```python
from build123d import *

# Parameters (mm, degrees)
SKETCH1_W                     = 444.26599996
SKETCH1_H                     = 47.498
BASE_FLANGE1_DEPTH            = 2.286
EDGE_FLANGE1_STRIP_W          = 11.144
EDGE_FLANGE1_STRIP_H          = 2.286
EDGE_FLANGE1_STRIP_CUT_DEPTH  = 25.4
EDGE_FLANGE1_RELIEF_W         = 12.287
EDGE_FLANGE1_RELIEF_H         = 1.143
EDGE_FLANGE1_RELIEF_CUT_DEPTH = 2.286
EDGE_FLANGE1_DEPTH            = 25.4
EDGE_FLANGE2_STRIP_W          = 11.144
EDGE_FLANGE2_STRIP_H          = 2.286
EDGE_FLANGE2_STRIP_CUT_DEPTH  = 25.4
EDGE_FLANGE2_RELIEF_W         = 12.287
EDGE_FLANGE2_RELIEF_H         = 1.143
EDGE_FLANGE2_RELIEF_CUT_DEPTH = 2.286
EDGE_FLANGE2_DEPTH            = 25.4
EDGE_FLANGE6_STRIP_W          = 11.144
EDGE_FLANGE6_STRIP_H          = 2.286
EDGE_FLANGE6_STRIP_CUT_DEPTH  = 444.26599996
EDGE_FLANGE6_DEPTH            = 444.26599996
SKETCH52_R                    = 3
CUT_EXTRUDE2_DEPTH            = 231.225159807
SKETCH53_R                    = 3
CUT_EXTRUDE3_DEPTH            = 450.771788169
SKETCH54_W                    = 20.32
SKETCH54_H                    = 3.286
CUT_EXTRUDE4_DEPTH            = 227.280796306
CUT_EXTRUDE6_DEPTH            = 227.280796306
CUT_EXTRUDE6_DEPTH_BACK       = 227.280796306
SKETCH57_W                    = 12.932384232
SKETCH57_H                    = 5.987852531
SKETCH57_W_2                  = 12.889095721
SKETCH57_H_2                  = 5.98785253
SKETCH57_W_3                  = 14.589217144
SKETCH57_H_3                  = 5.987852532
SKETCH57_W_4                  = 12.590694247
SKETCH57_H_4                  = 5.987852533
SKETCH57_W_5                  = 11.791285089
SKETCH57_H_5                  = 5.654723841


# Sheet-metal steps are written as plain solids
with BuildPart() as part:
    # Sketch1 → Base-Flange1 (new body)
    with BuildSketch(Plane.XY):
        Rectangle(SKETCH1_W, SKETCH1_H)
    extrude(amount=-BASE_FLANGE1_DEPTH)

    # Edge-Flange1 strip (across the edge) → Edge-Flange1 strip cut (cut)
    with BuildSketch(Plane(origin=(222.13299998, -12.7, 0), x_dir=(-1, 0, 0), z_dir=(0, 1, 0))):
        with Locations((-4.572, -1.143)):
            Rectangle(EDGE_FLANGE1_STRIP_W, EDGE_FLANGE1_STRIP_H)
    extrude(amount=EDGE_FLANGE1_STRIP_CUT_DEPTH, mode=Mode.SUBTRACT)

    # Edge-Flange1 relief (on the sheet) → Edge-Flange1 relief cut (cut)
    with BuildSketch(Plane(origin=(221.13299998, -12.7, 0), x_dir=(-1, 0, 0), z_dir=(0, 0, 1))):
        with Locations((-5.0005, 0.5715)):
            Rectangle(EDGE_FLANGE1_RELIEF_W, EDGE_FLANGE1_RELIEF_H)
        with Locations((-5.0005, -25.9715)):
            Rectangle(EDGE_FLANGE1_RELIEF_W, EDGE_FLANGE1_RELIEF_H)
    extrude(amount=-EDGE_FLANGE1_RELIEF_CUT_DEPTH, mode=Mode.SUBTRACT)

    # Edge-Flange1 section (across the edge) → Edge-Flange1 (add)
    with BuildSketch(Plane(origin=(222.13299998, -12.7, 0), x_dir=(-1, 0, 0), z_dir=(0, 1, 0))):
        with BuildLine():
            Line((-2.286, 1), (-2.286, 12.7))
            Line((-2.286, 12.7), (0, 12.7))
            Line((0, 12.7), (0, 1))
            ThreePointArc((0, 1), (0.292893219, 0.292893219), (1, 0))
            Line((1, 0), (1, -2.286))
            ThreePointArc((1, -2.286), (-1.323552883, -1.323552883), (-2.286, 1))
        make_face()
    extrude(amount=EDGE_FLANGE1_DEPTH)

    # Edge-Flange2 strip (across the edge) → Edge-Flange2 strip cut (cut)
    with BuildSketch(Plane(origin=(-222.13299998, 12.7, 0), x_dir=(1, 0, 0), z_dir=(0, -1, 0))):
        with Locations((-4.572, -1.143)):
            Rectangle(EDGE_FLANGE2_STRIP_W, EDGE_FLANGE2_STRIP_H)
    extrude(amount=EDGE_FLANGE2_STRIP_CUT_DEPTH, mode=Mode.SUBTRACT)

    # Edge-Flange2 relief (on the sheet) → Edge-Flange2 relief cut (cut)
    with BuildSketch(Plane(origin=(-221.13299998, 12.7, 0), x_dir=(1, 0, 0), z_dir=(0, 0, 1))):
        with Locations((-5.0005, 0.5715)):
            Rectangle(EDGE_FLANGE2_RELIEF_W, EDGE_FLANGE2_RELIEF_H)
        with Locations((-5.0005, -25.9715)):
            Rectangle(EDGE_FLANGE2_RELIEF_W, EDGE_FLANGE2_RELIEF_H)
    extrude(amount=-EDGE_FLANGE2_RELIEF_CUT_DEPTH, mode=Mode.SUBTRACT)

    # Edge-Flange2 section (across the edge) → Edge-Flange2 (add)
    with BuildSketch(Plane(origin=(-222.13299998, 12.7, 0), x_dir=(1, 0, 0), z_dir=(0, -1, 0))):
        with BuildLine():
            Line((-2.286, 1), (-2.286, 12.7))
            Line((-2.286, 12.7), (0, 12.7))
            Line((0, 12.7), (0, 1))
            ThreePointArc((0, 1), (0.292893219, 0.292893219), (1, 0))
            Line((1, 0), (1, -2.286))
            ThreePointArc((1, -2.286), (-1.323552883, -1.323552883), (-2.286, 1))
        make_face()
    extrude(amount=EDGE_FLANGE2_DEPTH)

    # Edge-Flange6 strip (across the edge) → Edge-Flange6 strip cut (cut)
    with BuildSketch(Plane(origin=(222.13299998, 23.749, 0), x_dir=(0, -1, 0), z_dir=(-1, 0, 0))):
        with Locations((-4.572, -1.143)):
            Rectangle(EDGE_FLANGE6_STRIP_W, EDGE_FLANGE6_STRIP_H)
    extrude(amount=EDGE_FLANGE6_STRIP_CUT_DEPTH, mode=Mode.SUBTRACT)

    # Edge-Flange6 section (across the edge) → Edge-Flange6 (add)
    with BuildSketch(Plane(origin=(222.13299998, 23.749, 0), x_dir=(0, -1, 0), z_dir=(-1, 0, 0))):
        with BuildLine():
            Line((-2.286, 1), (-2.286, 12.7))
            Line((-2.286, 12.7), (0, 12.7))
            Line((0, 12.7), (0, 1))
            ThreePointArc((0, 1), (0.292893219, 0.292893219), (1, 0))
            Line((1, 0), (1, -2.286))
            ThreePointArc((1, -2.286), (-1.323552883, -1.323552883), (-2.286, 1))
        make_face()
    extrude(amount=EDGE_FLANGE6_DEPTH)

    # Sketch52 → Cut-Extrude2 (cut, through all)
    with BuildSketch(Plane(origin=(0, 26.035, 0), x_dir=(1, 0, 0), z_dir=(0, 1, 0))):
        with Locations(Location((120.65, -6.85, 0), (0, 0, 270))):
            Circle(SKETCH52_R)
        with Locations(Location((-120.65, -6.85, 0), (0, 0, 270))):
            Circle(SKETCH52_R)
    extrude(amount=-CUT_EXTRUDE2_DEPTH, mode=Mode.SUBTRACT)

    # Sketch53 → Cut-Extrude3 (cut, through all)
    with BuildSketch(Plane(origin=(224.41899998, 0, 0), x_dir=(0, 0, -1), z_dir=(1, 0, 0))):
        with Locations((-6.85, 0)):
            Circle(SKETCH53_R)
    extrude(amount=-CUT_EXTRUDE3_DEPTH, mode=Mode.SUBTRACT)

    # Sketch54 → Cut-Extrude4 (cut, symmetric)
    with BuildSketch(Plane.XY):
        Polygon((222.13299998, 13.843), (222.13299998, 18.296), (201.81299998, 18.296), (201.81299998, 13.216), (219.98999998, 13.216), (219.98999998, 13.843), align=None)
        with Locations((211.97299998, 24.392)):
            Rectangle(SKETCH54_W, SKETCH54_H)
    cut_extrude4 = extrude(amount=CUT_EXTRUDE4_DEPTH, both=True, mode=Mode.SUBTRACT)

    # Mirror1: Cut-Extrude4 across plane
    add(cut_extrude4.mirror(Plane(origin=(0, 0, 0), x_dir=(0, 0, 1), z_dir=(1, 0, 0))), mode=Mode.SUBTRACT)

    # Sketch57 → Cut-Extrude6 (cut, two sides: drawn at the far end of the back side and taken through both)
    with BuildSketch(Plane.XY.offset(-CUT_EXTRUDE6_DEPTH_BACK)):
        with Locations((-85.29165905, -20.755073735)):
            Rectangle(SKETCH57_W, SKETCH57_H)
        with Locations((-187.864563379, -20.755073735)):
            Rectangle(SKETCH57_W_2, SKETCH57_H_2)
        with Locations((-5.245477464, -20.755073734)):
            Rectangle(SKETCH57_W_3, SKETCH57_H_3)
        with Locations((96.279485673, -20.755073734)):
            Rectangle(SKETCH57_W_4, SKETCH57_H_4)
        with Locations((176.220401529, -20.921638079)):
            Rectangle(SKETCH57_W_5, SKETCH57_H_5)
    extrude(amount=CUT_EXTRUDE6_DEPTH + CUT_EXTRUDE6_DEPTH_BACK, mode=Mode.SUBTRACT)


solid = part.part
```
Build history of the part. All positions in model axes, mm. A direction names the side the tool comes from. Round coordinates to 2 decimals unless told otherwise and drop trailing zeros. Loops run counter-clockwise (first coordinate to the right, second up) from the corner with the lowest first, then second, coordinate; pieces in that order, holes last.
Item 1: Two-plate mould, pull along X, no slides. Class faces 3 (the face through (-3, 0, 0)), 4 (the face through (-224.419, 3, 5)), 5 (the face through (3, 23.749, 7)): released by +X, released by -X, zero draft, split by the parting line, or undercut.
Item 2: Pin check, flat tips, straight feed: P1, Ø1.8, axis at y = 21.5, z = -1, coming from the -X side; P2, Ø2.5, axis at x = 209.5, z = -1.5, coming from the +Y side; P3, Ø2.5, axis at y = -21, z = -1.5, coming from the +X side. Stop position of each tip, or through.
Item 3: Saw through at A-A (z = 6.85). List the corners of the cut face in (x, y) (3 decimals), then the cut area to 3 significant figures.
Item 4: Which spindle directions (+Z, -Z, +X, -X, +Y, -Y) get a long thin tool onto all of the face, cutting with end or side? Do faces 1 (the face through (222.133, -3, 5.6)), 2 (the face through (-3, 0, -2.286)). Say none if no direction does.
Item 5: Saw through at B-B (x = 164). List the corners of the cut face in (y, z) (3 decimals).
Item 6: Drill centre lines: line 1 along X through (y, z) = (24.85, 6.85); line 2 along X through (y, z) = (-12.5, 10); line 3 along Y through (x, z) = (222.9, 6.85). Where is each one in solid material? Low to high.
Worked answers:
1. face 3: undercut
1. face 4: released by -X
1. face 5: zero draft
2. P1: stops at x = -222.13
2. P2: stops at y = 22.75
2. P3: stops at x = 222.13
3. outline: (-224.419, -12.7) - (-222.133, -12.7) - (-222.133, -3) - (-224.419, -3) - close; (-224.419, 3) - (-222.133, 3) - (-222.133, 12.7) - (-224.419, 12.7) - close; (-201.813, 23.749) - (-123.65, 23.749) - (-123.65, 26.035) - (-201.813, 26.035) - close; (-117.65, 23.749) - (117.65, 23.749) - (117.65, 26.035) - (-117.65, 26.035) - close; (123.65, 23.749) - (201.813, 23.749) - (201.813, 26.035) - (123.65, 26.035) - close; (222.133, -12.7) - (224.419, -12.7) - (224.419, -3) - (222.133, -3) - close; (222.133, 3) - (224.419, 3) - (224.419, 12.7) - (222.133, 12.7) - close
3. area: 984 mm2
4. face 1: +Z, +Y, -Y
4. face 2: -Z, +X, -X, +Y, -Y
5. outline: (-23.749, -2.286) - (22.749, -2.286) arc R3.286 ccw to (26.035, 1) - (26.035, 12.7) - (23.749, 12.7) - (23.749, 1) arc R1 cw to (22.749, 0) - (-23.749, 0) - close
6. line 1: x = -201.81 to -123.65, -117.65 to 117.65, 123.65 to 201.81
6. line 2: x = -224.42 to -222.13, 222.13 to 224.42
6. line 3: y = -12.7 to -3, 3 to 12.7
